```python
from build123d import *

# Parameters (mm, degrees)
F0_R      = 7.875
F2_R      = 6.1
F4_T      = -1
F5_R      = 3
F6_DEPTH  = 12.5
F7_R      = 1.225
F8_DEPTH  = 2.8
F9_W      = 2.908817606
F9_H      = 7.2918525926
F10_DEPTH = 20.9010001
F11_R     = 1


with BuildPart() as f3:
    # F0 (on Front) → F3 section 0
    with BuildSketch(Plane.XZ):
        Circle(F0_R)
    # F2 (on offset) → F3 section 1
    with BuildSketch(Plane.XZ.offset(20.9)):
        Circle(F2_R)
    loft()

    # F4
    f4_openings = [f3.faces().sort_by_distance(p)[0] for p in [
        (0, 0, 0),
    ]]
    offset(amount=F4_T, openings=f4_openings, kind=Kind.INTERSECTION)

    # F5 (on offset) → F6 (cut, symmetric)
    with BuildSketch(Plane.XZ.offset(20.9)):
        Circle(F5_R)
    extrude(amount=F6_DEPTH, both=True, mode=Mode.SUBTRACT)

    # F7 (on Right) → F8 (join, symmetric)
    with BuildSketch(Plane.YZ):
        with BuildLine():
            Line((-5.5590723408, -6.6040260717), (-5.5590723408, -14.9660339587))
            ThreePointArc((-5.5590723408, -14.9660339587), (-2.8090723408, -17.0962775531), (-0.0590723408, -14.9660339587))
            Line((-0.0590723408, -14.9660339587), (-0.0590723408, -7.0811193436))
            Line((-0.0590723408, -7.0811193436), (-5.5590723408, -6.6040260717))
        make_face()
        with Locations((-2.8090723408, -14.256124013)):
            Circle(F7_R, mode=Mode.SUBTRACT)
    extrude(amount=F8_DEPTH, both=True)

    # F9 (on offset) → F10 (cut, through all)
    with BuildSketch(Plane.XZ.offset(20.9)):
        with Locations((-0.016908803, -14.2587911789)):
            Rectangle(F9_W, F9_H)
    extrude(amount=-F10_DEPTH, mode=Mode.SUBTRACT)

    # F11
    f11_edges = [f3.edges().sort_by_distance(p)[0] for p in [
        (-6.1, -20.9, 0),
    ]]
    fillet(f11_edges, radius=F11_R)


solid = f3.part
```
The listing builds one solid part. Answer for the finished solid, in the listing's coordinates (mm). Coordinates: 2 decimals unless noted, no trailing zeros. Loops run counter-clockwise (first coordinate to the right, second up) from the corner with the lowest first, then second, coordinate; pieces in that order, holes last. Notation, with made-up numbers: (37, 32) -> (59, 32) arc R26 cw to (59, 70) -> close; hole circle Ø3 at (-27.75, -32). An arc over 180 degrees is marked (long way). Return JSON: item names as keys, results as strings. Group by question number.
(1) A cutting plane is placed at B-B on x = 0. Write down the section's boundary in (y, z) (3 decimals).
(2) Given pin 1 Ø4 at (y, z) = (-11.5, 0.5) entering from +X; pin 2 Ø4.5 at (x, z) = (-1, -10.5) entering from -Y; pin 3 Ø3 at (x, y) = (0, -18.5) entering from +Z; pin 4 Ø5 at (x, z) = (-1, -8) entering from +Y, each flat-ended and moving along its own axis, determine where each tip first touches the part or whether it passes through.
(3) A cutting plane is placed at D-D on x = 2.25. Count the separate pieces of the cut face and the enclosed holes in it, and give its area (3 significant figures).
(4) Find the intervals of material crossed by probe 1 along Y at (x, z) = (-2, -4.25); probe 2 along X at (y, z) = (-8.5, -3); probe 3 along Z at (x, y) = (0, -20.45), in increasing order. Write a range as from..to.
(5) A cutting plane is placed at A-A on y = -2.25. Write down the section's boundary in (x, z).
(6) A cutting plane is placed at C-C on y = -8.25. Write down the section's boundary in (x, z), and give its area (3 significant figures).
(7) Determine the mould class of faces 1 (the conical face through (3.8, -10.1, 5.9)), 2 (the cylindrical face through (2.128, -2.861, -17.096)), 3 (the flat face through (2.23, -19.9, -2.23)), 4 (the flat face through (2.23, -20.9, -2.23)) for opening direction Z: released by +Z, released by -Z, zero draft, split by the parting line, or undercut.
The answers:
{
 "1": {"outline": "(-20.9, -5.181) arc R1 ccw to (-19.985, -6.178) -> (-5.559, -7.403) -> (-5.559, -10.613) -> (-0.059, -10.613) -> (-0.059, -7.87) -> (0, -7.875) -> (0, -6.871) -> (-19.9, -5.181) -> (-19.9, -3) -> (-20.9, -3) -> close; (-20.9, 3) -> (-19.9, 3) -> (-19.9, 5.181) -> (0, 6.871) -> (0, 7.875) -> (-19.985, 6.178) arc R1 ccw to (-20.9, 5.181) -> close"},
 "2": {"pin 1": "stops at x = 7.06", "pin 2": "stops at y = -5.56", "pin 3": "stops at z = 6.43", "pin 4": "stops at y = 0"},
 "3": {"separate pieces": "2", "enclosed holes": "1", "area": "95.9 mm^2"},
 "4": {"probe 1": "y = -20.9..-19.9", "probe 2": "x = -6.49..-5.37, 5.37..6.49", "probe 3": "z = -6.02..-3, 3..6.02"},
 "5": {"outline": "(-2.8, -17.04) -> (-1.47, -17.04) -> (-1.47, -15.35) -> (-2.8, -15.35) -> close; (-2.8, -13.17) -> (-1.47, -13.17) -> (-1.47, -10.61) -> (1.44, -10.61) -> (1.44, -13.17) -> (2.8, -13.17) -> (2.8, -7.16) arc R7.68 ccw (long way) to (-2.8, -7.16) -> close; (1.44, -17.04) -> (2.8, -17.04) -> (2.8, -15.35) -> (1.44, -15.35) -> close; hole circle Ø13.36 at (0, 0)"},
 "6": {"outline": "circle Ø14.35 at (0, 0); hole circle Ø12.34 at (0, 0)", "area": "42.1 mm^2"},
 "7": {"face 1": "split by the parting line", "face 2": "released by -Z", "face 3": "undercut", "face 4": "zero draft"}
}
